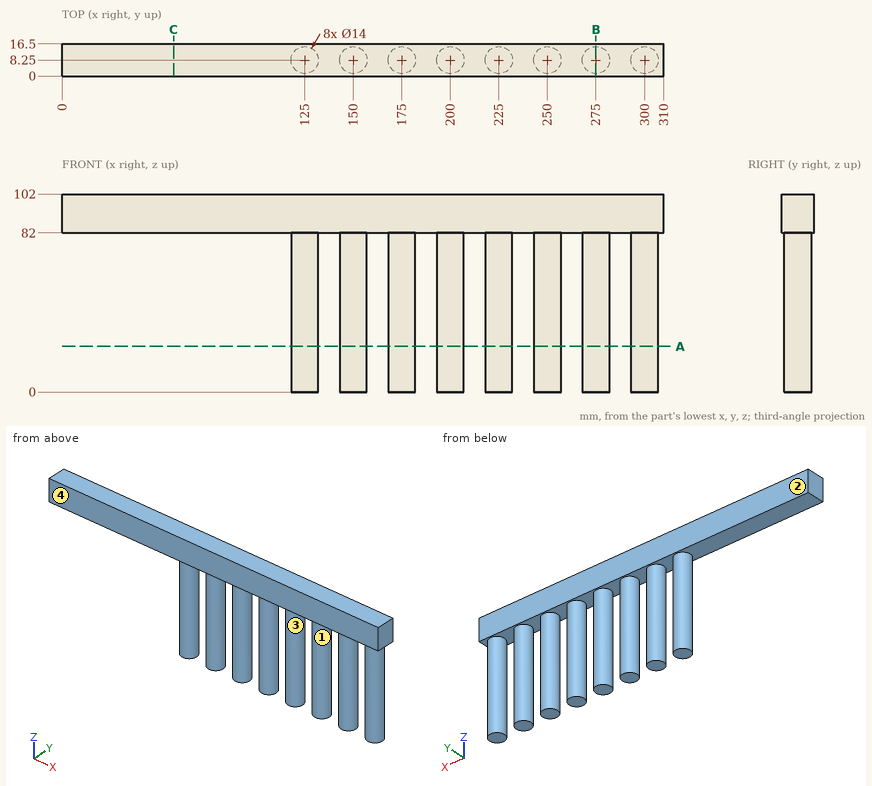
Answer from the drawing. Dimensions are ordinates in mm from the lowest x, y and z of the part. A direction names the side the tool comes from. Give positions to 0.01 mm unless a question says otherwise; leave off trailing zeros. Write each loop counter-clockwise with the first axis right and the second up, starting at its lowest first coordinate (ties: lowest second). Pieces come first, ordered by that corner, then holes. Notation, with made-up numbers: (46.25, 7.5) -> (55.25, 7.5) arc R16 ccw to (55.25, 13.5) -> close; hole circle Ø3 at (28.5, 34.5). An arc over 180 degrees is marked (long way). Use a Markdown table: item, result.
(1) Flat-ended cylindrical pins translate along their axes: P1, Ø1, axis at y = 14, z = 74, coming from the +X side; P2, Ø5, axis at x = 85, y = 9.5, coming from the -Z side; P3, Ø2, axis at x = 171.5, z = 76, coming from the -Y side; P4, Ø6, axis at x = 164.5, z = 70.5, coming from the -Y side. Find the tip coordinate at first contact, or state that the pin passes through.
Return value:
| item | result |
|---|---|
| P1 | x = 304.63 |
| P2 | z = 82 |
| P3 | y = 1.71 |
| P4 | through |
(2) Find the intervals of material crossed by probe 1 along Z at (x, y) = (53.5, 2); probe 2 along Y at (x, z) = (222, 17.5); probe 3 along Y at (x, z) = (222.5, 33.5), in increasing order. Write a range as from..to.
Return value:
| item | result |
|---|---|
| probe 1 | 82..102 |
| probe 2 | 1.93..14.57 |
| probe 3 | 1.71..14.79 |
(3) Section B-B, the plane x = 275 is taken. Determine the outline of the cut face in (y, z).
Return value:
| item | result |
|---|---|
| outline | (0, 82) -> (1.25, 82) -> (1.25, 0) -> (15.25, 0) -> (15.25, 82) -> (16.5, 82) -> (16.5, 102) -> (0, 102) -> close |
(4) Determine the mould class of the marked faces 3 and 4 for opening direction X: released by +X, released by -X, zero draft, split by the parting line, or undercut.
Return value:
| item | result |
|---|---|
| face 3 | undercut |
| face 4 | zero draft |
(5) Section A-A, the plane z = 23.5 is taken. Determine the outline of the cut face in (x, y).
Return value:
| item | result |
|---|---|
| outline | circle Ø14 at (125, 8.25); circle Ø14 at (150, 8.25); circle Ø14 at (175, 8.25); circle Ø14 at (200, 8.25); circle Ø14 at (225, 8.25); circle Ø14 at (250, 8.25); circle Ø14 at (275, 8.25); circle Ø14 at (300, 8.25) |
(6) Section C-C, the plane x = 57.5 is taken. Determine the outline of the cut face in (y, z), then the cut area to 3 significant figures.
Return value:
| item | result |
|---|---|
| outline | (0, 82) -> (16.5, 82) -> (16.5, 102) -> (0, 102) -> close |
| area | 330 mm2 |
(7) For the marked faces 1 and 2, determine the directions among +Z, -Z, +X, -X, +Y, -Y from which every point of the face is accessible in a straight line to the end or side of a thin tool.
Return value:
| item | result |
|---|---|
| face 1 | -Z |
| face 2 | +Z, -Z, +X, -X, +Y |
